from build123d import *

# Parameters (mm, degrees)
IZIM1_W                     = 172.5
IZIM1_H                     = 103.4
IZIM1_W_2                   = 165
IZIM1_H_2                   = 98.4
Y_KSEKLIK_EKSTR_ZYON1_DEPTH = 6
Y_KSEKLIK_EKSTR_ZYON2_DEPTH = 1
IZIM3_R                     = 2.25
Y_KSEKLIK_EKSTR_ZYON3_DEPTH = 7


with BuildPart() as part:
    # Çizim1 → Yükseklik-Ekstrüzyon1 (new body)
    with BuildSketch(Plane(origin=(0, 0, 0), x_dir=(0, 1, 0), z_dir=(0, 0, 1))):
        with Locations((47.811428221, -21.27957211)):
            Rectangle(IZIM1_W, IZIM1_H)
        with Locations((46.561428221, -21.27957211)):
            Rectangle(IZIM1_W_2, IZIM1_H_2, mode=Mode.SUBTRACT)
    extrude(amount=Y_KSEKLIK_EKSTR_ZYON1_DEPTH)

    # Çizim2 → Yükseklik-Ekstrüzyon2 (add)
    with BuildSketch(Plane.XY.offset(6)):
        Polygon((-30.42042789, 54.561428221), (-30.42042789, 134.061428221), (72.97957211, 134.061428221), (72.97957211, -38.438571779), (-30.42042789, -38.438571779), (-30.42042789, 24.561428221), align=None)
        with BuildLine():
            Line((-27.92042789, 24.561428221), (-6.52042789, 24.561428221))
            ThreePointArc((-6.52042789, 24.561428221), (-5.813321109, 24.85432144), (-5.52042789, 25.561428221))
            Line((-5.52042789, 25.561428221), (-5.52042789, 53.561428221))
            ThreePointArc((-5.52042789, 53.561428221), (-5.813321109, 54.268535002), (-6.52042789, 54.561428221))
            Line((-6.52042789, 54.561428221), (-27.92042789, 54.561428221))
            Line((-27.92042789, 54.561428221), (-27.92042789, 24.561428221))
        make_face(mode=Mode.SUBTRACT)
    extrude(amount=Y_KSEKLIK_EKSTR_ZYON2_DEPTH)

    # Çizim3 → Yükseklik-Ekstrüzyon3 (add)
    # profile 1 of 4: a face of its own
    with BuildSketch(Plane(origin=(0, 0, 0), x_dir=(0, 1, 0), z_dir=(0, 0, 1))):
        with BuildLine():
            Line((-38.438571779, 30.42042789), (-47.938571779, 30.42042789))
            Line((-47.938571779, 30.42042789), (-47.938571779, 23.42042789))
            ThreePointArc((-47.938571779, 23.42042789), (-47.206338732, 21.652660937), (-45.438571779, 20.92042789))
            Line((-45.438571779, 20.92042789), (-38.438571779, 20.92042789))
            Line((-38.438571779, 20.92042789), (-38.438571779, 30.42042789))
        make_face()
        with Locations(Location((-43.188571779, 25.67042789, 0), (0, 0, 90))):
            Circle(IZIM3_R, mode=Mode.SUBTRACT)
    # profile 2 of 4: a face of its own
    with BuildSketch(Plane(origin=(0, 0, 0), x_dir=(0, 1, 0), z_dir=(0, 0, 1))):
        with BuildLine():
            Line((-38.438571779, -61.85378906), (-45.438571779, -61.85378906))
            ThreePointArc((-45.438571779, -61.85378906), (-47.206338732, -62.586022107), (-47.938571779, -64.35378906))
            Line((-47.938571779, -64.35378906), (-47.938571779, -72.97957211))
            Line((-47.938571779, -72.97957211), (-38.438571779, -72.97957211))
            Line((-38.438571779, -72.97957211), (-38.438571779, -61.85378906))
        make_face()
        with Locations(Location((-43.188571779, -67.416680585, 0), (0, 0, 90))):
            Circle(IZIM3_R, mode=Mode.SUBTRACT)
    # profile 3 of 4: a face of its own
    with BuildSketch(Plane(origin=(0, 0, 0), x_dir=(0, 1, 0), z_dir=(0, 0, 1))):
        with BuildLine():
            Line((142.961428221, 30.42042789), (134.061428221, 30.42042789))
            Line((134.061428221, 30.42042789), (134.061428221, 20.186573321))
            Line((134.061428221, 20.186573321), (140.461428221, 20.186573321))
            ThreePointArc((140.461428221, 20.186573321), (142.229195174, 20.918806368), (142.961428221, 22.686573321))
            Line((142.961428221, 22.686573321), (142.961428221, 30.42042789))
        make_face()
        with Locations(Location((138.511428221, 25.303500605, 0), (0, 0, 90))):
            Circle(IZIM3_R, mode=Mode.SUBTRACT)
    # profile 4 of 4: a face of its own
    with BuildSketch(Plane(origin=(0, 0, 0), x_dir=(0, 1, 0), z_dir=(0, 0, 1))):
        with BuildLine():
            Line((140.461428221, -63.47957211), (134.061428221, -63.47957211))
            Line((134.061428221, -63.47957211), (134.061428221, -72.97957211))
            Line((134.061428221, -72.97957211), (142.961428221, -72.97957211))
            Line((142.961428221, -72.97957211), (142.961428221, -65.97957211))
            ThreePointArc((142.961428221, -65.97957211), (142.229195174, -64.211805157), (140.461428221, -63.47957211))
        make_face()
        with Locations(Location((138.511428221, -68.22957211, 0), (0, 0, 90))):
            Circle(IZIM3_R, mode=Mode.SUBTRACT)
    extrude(amount=Y_KSEKLIK_EKSTR_ZYON3_DEPTH)


solid = part.part
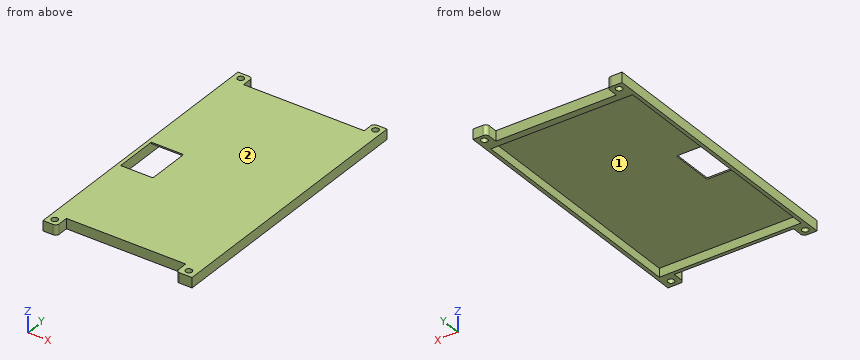
Verification items for the finished model (mm, model axes). Face numbers are marked on the shaded views. Give positions to 0.01 mm unless a question says otherwise; leave off trailing zeros. Write each loop counter-clockwise with the first axis right and the second up, starting at its lowest first coordinate (ties: lowest second). Pieces come first, ordered by that corner, then holes.
(1) Cross-section at A-A (y = 31). Enter the section's corners in (x, z).
(2) Cross-section at B-B (x = -10.5). Enter the section's corners in (y, z).
(3) Cross-section at D-D (x = 49.5). Enter the section's corners in (y, z).
(4) Gauge pin test, flat ends, axial feed: pin 1 (3.5 mm diameter, centred on x = 4, z = 5, fed in from -Y); pin 2 (0.8 mm diameter, centred on x = -16.5, z = 6.5, fed in from +Y); pin 3 (4 mm diameter, centred on x = -0.5, y = 75.5, fed in from -Z). Record the tip position at first contact, or that the pin passes through.
(5) Material ranges on line 1 (Y direction, x = 11, z = 2.5); line 2 (X direction, y = 81, z = 1.5); line 3 (Y direction, x = 67.5, z = 2.5), recorded low to high.
(6) Cross-section at C-C (z = 2.75). Enter the section's corners in (x, y), plus the area to 3 significant figures.
(7) Mould release check, pull along Y, two halves, no side actions. Record for the marked faces 1 and 2: +Y half, -Y half, draft (parallel to the pull), parting line (faces both ways), or undercut.
Worked out:
1. outline: (-30.42, 0) - (-27.92, 0) - (-27.92, 7) - (-30.42, 7) - close; (-5.52, 6) - (70.48, 6) - (70.48, 0) - (72.98, 0) - (72.98, 7) - (-5.52, 7) - close
2. outline: (-38.44, 0) - (-35.94, 0) - (-35.94, 6) - (24.56, 6) - (24.56, 7) - (-38.44, 7) - close; (54.56, 6) - (129.06, 6) - (129.06, 0) - (134.06, 0) - (134.06, 7) - (54.56, 7) - close
3. outline: (-38.44, 0) - (-35.94, 0) - (-35.94, 6) - (129.06, 6) - (129.06, 0) - (134.06, 0) - (134.06, 7) - (-38.44, 7) - close
4. pin 1: stops at y = -38.44
4. pin 2: stops at y = 134.06
4. pin 3: stops at z = 6
5. line 1: y = -38.44 to -35.94, 129.06 to 134.06
5. line 2: x = -30.42 to -27.92, 70.48 to 72.98
5. line 3: y = -47.94 to -45.44, -40.94 to -35.94, 129.06 to 136.38, 140.64 to 142.96
6. outline: (-30.42, -47.94) - (-23.42, -47.94) arc R2.5 ccw to (-20.92, -45.44) - (-20.92, -38.44) - (61.85, -38.44) - (61.85, -45.44) arc R2.5 ccw to (64.35, -47.94) - (72.98, -47.94) - (72.98, 142.96) - (65.98, 142.96) arc R2.5 ccw to (63.48, 140.46) - (63.48, 134.06) - (-20.19, 134.06) - (-20.19, 140.46) arc R2.5 ccw to (-22.69, 142.96) - (-30.42, 142.96) - close; hole circle Ø4.5 at (-25.67, -43.19); hole (-27.92, -35.94) - (70.48, -35.94) - (70.48, 129.06) - (-27.92, 129.06) - close; hole circle Ø4.5 at (-25.3, 138.51); hole circle Ø4.5 at (67.42, -43.19); hole circle Ø4.5 at (68.23, 138.51)
6. area: 1,900 mm2
7. face 1: undercut
7. face 2: draft
